Drawing for the job (mm, zero at the part's lowest x, y, z). A direction names the side the tool comes from. Round coordinates to 2 decimals unless told otherwise and drop trailing zeros. Loops run counter-clockwise (first coordinate to the right, second up) from the corner with the lowest first, then second, coordinate; pieces in that order, holes last. Notation, with made-up numbers: M -36.5,66 L -19.5,66 A27 cw -19.5,86 Z; hole C 61,36 d8. An arc over 180 degrees is marked long. Answer in a Markdown table with one row per item.
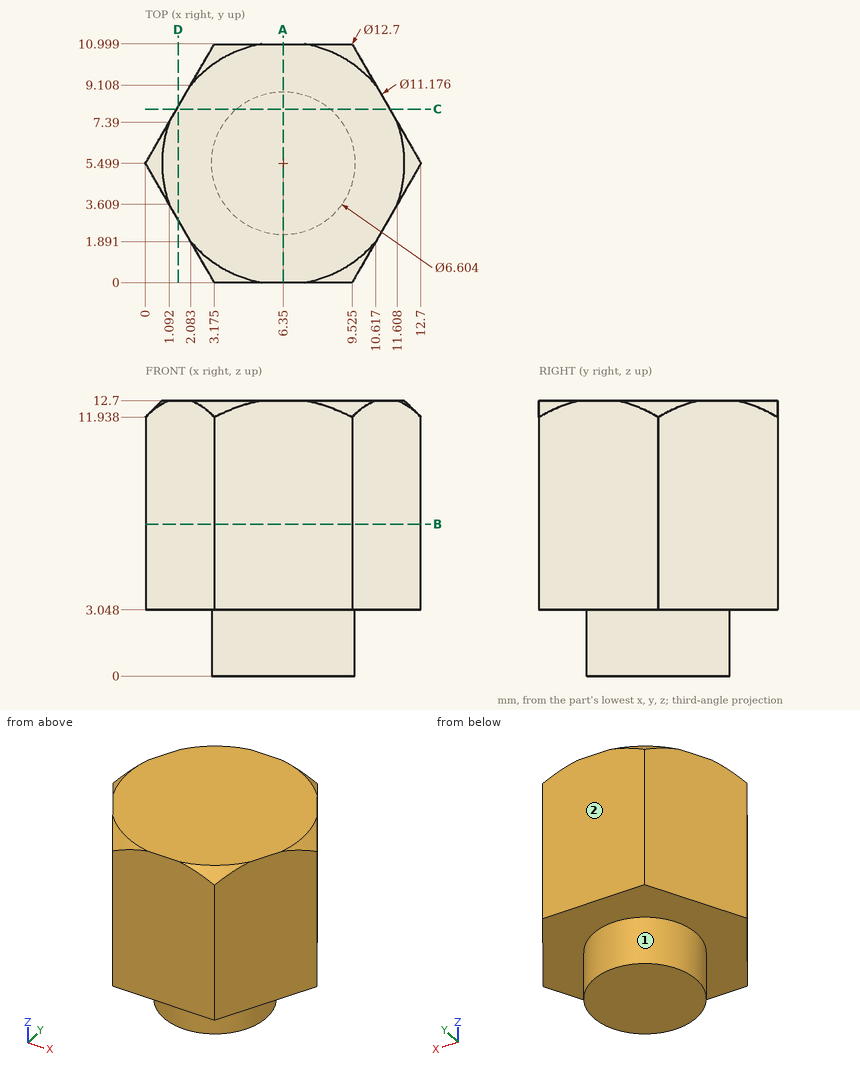
1. Saw through at A-A (x = 6.35). Write the cut outline in (y, z), and give its area (3 significant figures).
Verdict:
| item | result |
|---|---|
| outline | M 0,3.05 L 2.2,3.05 L 2.2,0 L 8.8,0 L 8.8,3.05 L 11,3.05 L 11,12.7 L 0,12.7 Z |
| area | 126 mm² |
2. Saw through at B-B (z = 7). Write the cut outline in (x, y) (1 decimal).
Verdict:
| item | result |
|---|---|
| outline | M 0,5.5 L 3.2,0 L 9.5,0 L 12.7,5.5 L 9.5,11 L 3.2,11 Z |
3. Saw through at D-D (x = 1.5). Write the cut outline in (y, z).
Verdict:
| item | result |
|---|---|
| outline | M 2.9,3.05 L 8.1,3.05 L 8.1,12.7 L 2.9,12.7 Z |
4. Saw through at C-C (y = 8). Write the cut outline in (x, z).
Verdict:
| item | result |
|---|---|
| outline | M 1.44,3.05 L 4.19,3.05 L 4.19,0 L 8.51,0 L 8.51,3.05 L 11.26,3.05 L 11.26,12.7 L 1.44,12.7 Z |
5. Pin check, flat tips, straight feed: pin 1 (3 mm diameter, centred on y = 8.5, z = 6, fed in from +X); pin 2 (5 mm diameter, centred on x = 10.5, z = 5.5, fed in from +Y). Stop position of each tip, or through.
Verdict:
| item | result |
|---|---|
| pin 1 | stops at x = 11.83 |
| pin 2 | stops at y = 11 |
6. Wall check: probe 1 along Z at (x, y) = (9, 9.25); probe 2 along X at (y, z) = (4, 3.25) (1 decimal); probe 3 along X at (y, z) = (8.5, 6.5). Give the ranges that are in metal, low to high.
Verdict:
| item | result |
|---|---|
| probe 1 | z = 3.05 to 12.7 |
| probe 2 | x = 0.9 to 11.8 |
| probe 3 | x = 1.73 to 10.97 |
7. Tool access for the marked faces 1 and 2: list every direction of +Z, -Z, +X, -X, +Y, -Y with a clear straight run to the whole face (end or side of a thin tool).
Verdict:
| item | result |
|---|---|
| face 1 | -Z |
| face 2 | +Z, -Z, +X, -X, +Y |
